Could you check a few things on this model? Use its own coordinates, in mm. Face numbers are marked on the shaded views. Coordinates: 2 decimals unless noted, no trailing zeros. Loops run counter-clockwise (first coordinate to the right, second up) from the corner with the lowest first, then second, coordinate; pieces in that order, holes last. Notation, with made-up numbers: (-0.5, 26.25) -> (22.5, 26.25) arc R14 cw to (22.5, 40.25) -> close; hole circle Ø2 at (15, -20). An arc over 180 degrees is marked (long way). One line per question, with ' | ' between items.
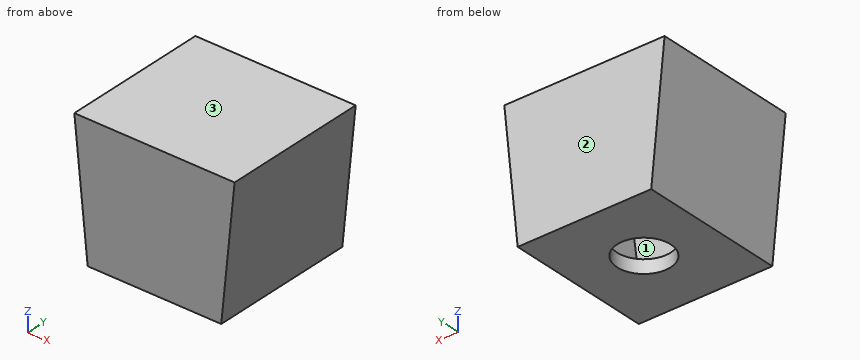
from build123d import *

# Parameters (mm, degrees)
F1_DEPTH = 225
F4_DEPTH = 25
F6_DEPTH = 25
F7_R     = 50
F8_DEPTH = 25


with BuildPart() as f1:
    # F0 (on Front) → F1 (new body)
    with BuildSketch(Plane.XZ):
        Polygon((-125, -125), (125, -125), (150, 125), (-150, 125), align=None)
        Polygon((125, 100), (100, -100), (-100, -100), (-125, 100), align=None, mode=Mode.SUBTRACT)
    extrude(amount=F1_DEPTH)

    # F3 (on face) + F2 (on face) → F4 (join)
    with BuildSketch(Plane.XZ.offset(225)):
        Polygon((125, -125), (150, 125), (-150, 125), (-125, -125), align=None)
    with BuildSketch(Plane.XZ.offset(225)):
        Polygon((-150, 125), (-125, -125), (125, -125), (150, 125), align=None)
        Polygon((-100, -100), (-125, 100), (125, 100), (100, -100), align=None, mode=Mode.SUBTRACT)
    extrude(amount=F4_DEPTH)

    # F5 (on face) → F6 (join)
    with BuildSketch(Plane(origin=(0, 0, 0), x_dir=(-1, 0, 0), z_dir=(0, 1, 0))):
        Polygon((125, -125), (150, 125), (-150, 125), (-125, -125), align=None)
    extrude(amount=F6_DEPTH)

    # F7 (on face) → F8 (cut)
    with BuildSketch(Plane(origin=(0, 0, -125), x_dir=(1, 0, 0), z_dir=(0, 0, -1))):
        with Locations((0, 110)):
            Circle(F7_R)
    extrude(amount=-F8_DEPTH, mode=Mode.SUBTRACT)


solid = f1.part
1) If we section it at B-B on z = -68: Please give me the cut outline in (x, y), and give its area (3 significant figures).
Data:
outline: (-130.7, -250) -> (130.7, -250) -> (130.7, 25) -> (-130.7, 25) -> close; hole (-104, -225) -> (104, -225) -> (104, 0) -> (-104, 0) -> close | area: 25,100 mm²
2) If we section it at D-D on x = 0: Please give me the cut outline in (y, z).
Data:
outline: (-250, -125) -> (-160, -125) -> (-160, -100) -> (-225, -100) -> (-225, 100) -> (0, 100) -> (0, -100) -> (-60, -100) -> (-60, -125) -> (25, -125) -> (25, 125) -> (-250, 125) -> close
3) If we section it at A-A on y = -183.5: Please give me the cut outline in (x, z).
Data:
outline: (-150, 125) -> (-125, -125) -> (125, -125) -> (150, 125) -> close; hole (-125, 100) -> (-100, -100) -> (100, -100) -> (125, 100) -> close
4) We'd pull the mould along Y, two halves only. Please class the marked faces 1, 2 and 3: pulls with the +Y half, pulls with the -Y half, needs draft (parallel to the pull), parting line crosses it, or undercut.
Data:
face 1: undercut | face 2: pulls with the +Y half | face 3: needs draft
5) I need wall thicknesses on line 1 along Y through (x, z) = (-74, 21.5); line 2 along Z through (x, y) = (-90, -136.5); line 3 along Y through (x, z) = (0, -106). Which ranges of each line are inside material? Lowest first, please. Write a range as from..to.
Data:
line 1: -250..-225, 0..25 | line 2: -125..-100, 100..125 | line 3: -250..-160, -60..25
6) If we section it at C-C on y = -110: Please give me the cut outline in (x, z), and give its area (4 significant figures).
Data:
outline: (-150, 125) -> (-125, -125) -> (-50, -125) -> (-50, -100) -> (-100, -100) -> (-125, 100) -> (125, 100) -> (100, -100) -> (50, -100) -> (50, -125) -> (125, -125) -> (150, 125) -> close | area: 21,250 mm²
7) I'm going to push flat-ended pins straight in: pin 1 Ø5 at (y, z) = (-86.5, -57) entering from +X; pin 2 Ø1 at (y, z) = (-62, 31.5) entering from -X; pin 3 Ø2 at (y, z) = (-133.5, 12) entering from -X. Where does each tip first touch, or does it pass through?
Data:
pin 1: x = 132.05 | pin 2: x = -140.7 | pin 3: x = -138.8
